The figure shows three views and two pictorial views of one solid part (mm, origin at its lowest corner). Answer the questions. Round coordinates to 2 decimals unless told otherwise and drop trailing zeros. Write each loop counter-clockwise with the first axis right and the second up, starting at its lowest first coordinate (ties: lowest second). Pieces come first, ordered by that corner, then holes.
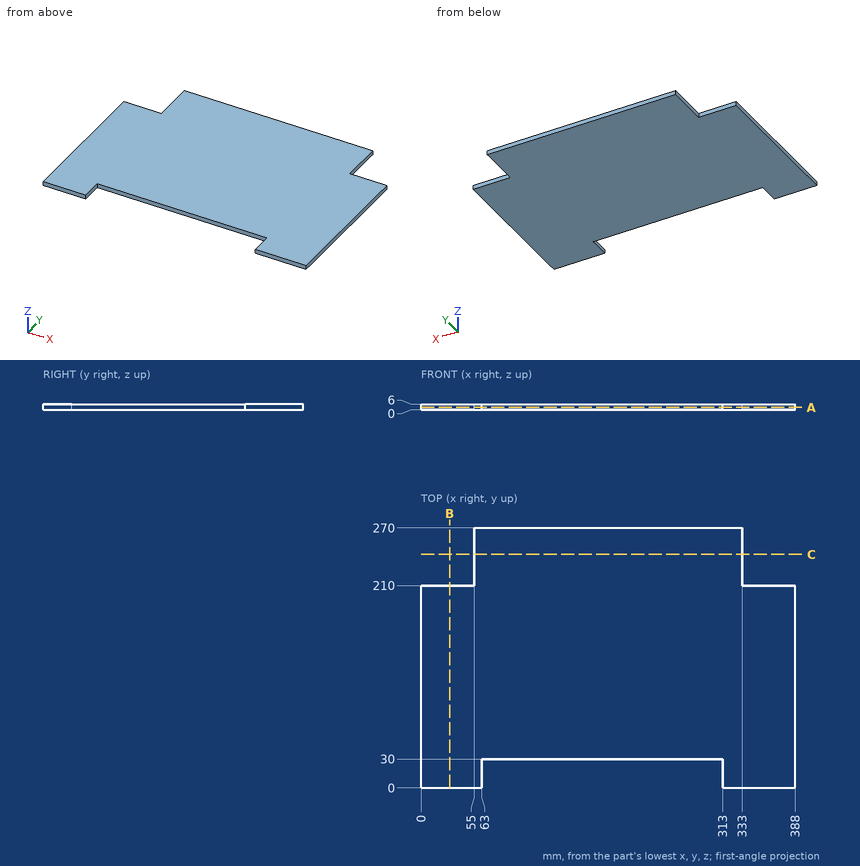
Q1. Flat-ended cylindrical pins translate along their axes: pin 1 Ø3 at (x, z) = (29.5, 1.5) entering from +Y; pin 2 Ø3 at (y, z) = (252, 2) entering from -X; pin 3 Ø2 at (x, y) = (328.5, 227) entering from -Z; pin 4 Ø1.8 at (x, z) = (167.5, 3) entering from -Y. Find the tip coordinate at first contact, or state that the pin passes through.
Verdict:
pin 1: stops at y = 210
pin 2: stops at x = 55
pin 3: stops at z = 0
pin 4: stops at y = 30
Q2. Section B-B (x = 29.5) is taken. Determine the outline of the cut face in (y, z).
Verdict:
outline: (0, 0) - (210, 0) - (210, 6) - (0, 6) - close
Q3. Straight lines are drawn through the part: probe 1 along Y at (x, z) = (19, 3.05); probe 2 along Y at (x, z) = (139, 0.3); probe 3 along X at (y, z) = (259.5, 2.85). For each, find the intervals that lie inside material, in ascending order.
Verdict:
probe 1: y = 0 to 210
probe 2: y = 30 to 270
probe 3: x = 55 to 333
Q4. Section A-A (z = 2.4) is taken. Determine the outline of the cut face in (x, y), then the cut area to 3 significant figures.
Verdict:
outline: (0, 0) - (63, 0) - (63, 30) - (313, 30) - (313, 0) - (388, 0) - (388, 210) - (333, 210) - (333, 270) - (55, 270) - (55, 210) - (0, 210) - close
area: 90,700 mm2
Q5. Section C-C (y = 242.5) is taken. Determine the outline of the cut face in (x, z).
Verdict:
outline: (55, 0) - (333, 0) - (333, 6) - (55, 6) - close
